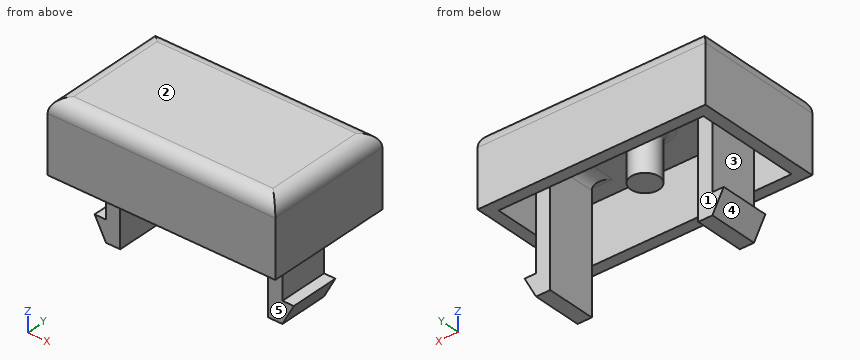
from build123d import *

# Parameters (mm, degrees)
SKETCH036_W     = 16
SKETCH036_H     = 9
PAD021_DEPTH    = 5
SKETCH037_W     = 14.4
SKETCH037_H     = 7.4
POCKET013_DEPTH = 4
SKETCH038_W     = 1
SKETCH038_H     = 3.5
PAD022_DEPTH    = 9
PAD023_DEPTH    = 3.5
SKETCH041_R     = 1
PAD025_DEPTH    = 3.4
FILLET002_R     = 1
FILLET007_R     = 0.7
FILLET011_R     = 0.8


with BuildPart() as part:
    # Sketch036 → Pad021 (new body)
    with BuildSketch(Plane.XY):
        Rectangle(SKETCH036_W, SKETCH036_H)
    extrude(amount=PAD021_DEPTH)

    # Sketch037 (on Face5 of Pad021) → Pocket013 (cut)
    with BuildSketch(Plane(origin=(0, 0, 0), x_dir=(1, 0, 0), z_dir=(0, 0, -1))):
        Rectangle(SKETCH037_W, SKETCH037_H)
    extrude(amount=-POCKET013_DEPTH, mode=Mode.SUBTRACT)

    # Sketch038 (on Face11 of Pocket013) → Pad022 (join)
    with BuildSketch(Plane(origin=(0, 0, 4), x_dir=(1, 0, 0), z_dir=(0, 0, -1))):
        with Locations((-5.7, 0)):
            Rectangle(SKETCH038_W, SKETCH038_H)
        with Locations((5.7, 0)):
            Rectangle(SKETCH038_W, SKETCH038_H)
    extrude(amount=PAD022_DEPTH)

    # Sketch039 (on Face17 of Pad022) → Pad023 (join)
    with BuildSketch(Plane(origin=(0, 1.75, 0), x_dir=(-1, 0, 0), z_dir=(0, 1, 0))):
        Polygon((-6.2, -3.5), (-7, -3.5), (-6.2, -5), align=None)
        Polygon((6.2, -3.5), (7, -3.5), (6.2, -5), align=None)
    extrude(amount=-PAD023_DEPTH)

    # Sketch041 (on Face11 of Pad023) → Pad025 (join)
    with BuildSketch(Plane(origin=(0, 0, 4), x_dir=(1, 0, 0), z_dir=(0, 0, -1))):
        Circle(SKETCH041_R)
    extrude(amount=PAD025_DEPTH)

    # Fillet002
    fillet002_edges = [part.edges().sort_by_distance(p)[0] for p in [
        (0, 4.5, 5),
        (-8, 0, 5),
        (0, -4.5, 5),
        (8, 0, 5),
    ]]
    fillet(fillet002_edges, radius=FILLET002_R)

    # Fillet007
    fillet007_edges = [part.edges().sort_by_distance(p)[0] for p in [
        (-1, 0, 4),
    ]]
    fillet(fillet007_edges, radius=FILLET007_R)

    # Fillet011
    fillet011_edges = [part.edges().sort_by_distance(p)[0] for p in [
        (5.2, 0, 4),
        (5.7, 1.75, 4),
        (6.2, 0, 4),
        (5.7, -1.75, 4),
        (-5.7, -1.75, 4),
        (-6.2, 0, 4),
        (-5.2, 0, 4),
        (-5.7, 1.75, 4),
    ]]
    fillet(fillet011_edges, radius=FILLET011_R)


with BuildPart() as part_1:
    # Body008 placement: moved
    add(part.part.moved(Location((-33, -44, 15))))


with BuildPart() as part_2:
    # Clone003 placement: moved
    add(part_1.part.moved(Location((0, 0, 4))))


with BuildPart() as part_3:
    # Body012 placement: moved
    add(part_2.part.moved(Location((68, 0, -4))))


solid = part_3.part
Design review of the part built by this model. Coordinates are the model's own, in mm. Face numbers are marked on the shaded views. A direction names the side the tool comes from. Coordinates: 2 decimals unless noted, no trailing zeros. Loops run counter-clockwise (first coordinate to the right, second up) from the corner with the lowest first, then second, coordinate; pieces in that order, holes last.
Item 1: Add section B-B (z = 13). Write out the cut boundary in (x, y), and give its area (3 significant figures).
Completed:
outline: (28.8, -45.75) - (29.8, -45.75) - (29.8, -42.25) - (28.8, -42.25) - close; (40.2, -45.75) - (41.2, -45.75) - (41.2, -42.25) - (40.2, -42.25) - close
area: 7.00 mm2
Item 2: Wall thickness on L1, parallel to Y at x = 40.25, z = 18.25; L2, parallel to X at y = -40.5, z = 15.25; L3, parallel to X at y = -45.25, z = 18.5: over which ranges is each line inside the solid? List them lowest first.
Completed:
L1: y = -48.5 to -47.7, -45.75 to -42.25, -40.3 to -39.5
L2: x = 27 to 27.8, 42.2 to 43
L3: x = 27 to 27.8, 28.74 to 29.86, 40.14 to 41.26, 42.2 to 43
Item 3: Draft analysis for pull direction Z (two halves, no side actions). For the marked faces 1, 2 and 3, state which applies: pulls with the +Z half, pulls with the -Z half, needs draft (parallel to the pull), parting line crosses it, or undercut.
Completed:
face 1: needs draft
face 2: pulls with the +Z half
face 3: undercut
Item 4: For the marked faces 4 and 5, list the 3-axis set-ups (+Z, -Z, +X, -X, +Y, -Y) from which the entire face can be reached by the end or side of a thin tool; tool diameter is ignored.
Completed:
face 4: -Z, -X, +Y, -Y
face 5: -Z
Item 5: Add section A-A (z = 18). Write out the cut boundary in (x, y), and give its area (3 significant figures).
Completed:
outline: (27, -48.5) - (43, -48.5) - (43, -39.5) - (27, -39.5) - close; (28.8, -45.75) - (29.8, -45.75) - (29.8, -42.25) - (28.8, -42.25) - close; circle Ø2 at (35, -44); (40.2, -45.75) - (41.2, -45.75) - (41.2, -42.25) - (40.2, -42.25) - close; hole (27.8, -47.7) - (42.2, -47.7) - (42.2, -40.3) - (27.8, -40.3) - close
area: 47.6 mm2
Item 6: Clearance check with flat-ended pins moving along their axes: pin 1 (1 mm diameter, centred on x = 35, y = -43.5, fed in from -Z); pin 2 (1 mm diameter, centred on y = -44, z = 12.5, fed in from +X); pin 3 (1 mm diameter, centred on y = -43, z = 14, fed in from -X). State where each tip first meets the part, or that it passes through.
Completed:
pin 1: stops at z = 15.6
pin 2: stops at x = 41.2
pin 3: stops at x = 28.8
Item 7: Add section C-C (x = 28.5). Write out the cut boundary in (y, z).
Completed:
outline: (-48.5, 15) - (-47.7, 15) - (-47.7, 19) - (-46.55, 19) arc R0.8 cw to (-46.05, 18.82) - (-41.95, 18.82) arc R0.8 cw to (-41.45, 19) - (-40.3, 19) - (-40.3, 15) - (-39.5, 15) - (-39.5, 19) arc R1 ccw to (-40.5, 20) - (-47.5, 20) arc R1 ccw to (-48.5, 19) - close; (-45.75, 10.56) - (-42.25, 10.56) - (-42.25, 11.5) - (-45.75, 11.5) - close
Item 8: Add section D-D (y = -47). Write out the cut boundary in (x, z), and give its area (3 significant figures).
Completed:
outline: (27, 15) - (27.8, 15) - (27.8, 19) - (42.2, 19) - (42.2, 15) - (43, 15) - (43, 19) arc R1 ccw to (42, 20) - (28, 20) arc R1 ccw to (27, 19) - close
area: 22.0 mm2
